Job drawing, mm, ordinate dimensions from the low corner. One solid piece. A direction names the side the tool comes from. Coordinates: 2 decimals unless noted, no trailing zeros. Order: outer loops, then holes, each group sorted by start corner. A loop starts at its lowest first (then second) coordinate and runs counter-clockwise, first axis right, second up. Notation, with made-up numbers: (56.25, 6.5) - (109.25, 6.5) arc R20 cw to (109.25, 25.5) - close; hole circle Ø6 at (-1.75, 29). An arc over 180 degrees is marked (long way). Return JSON: item names as keys, results as strings.
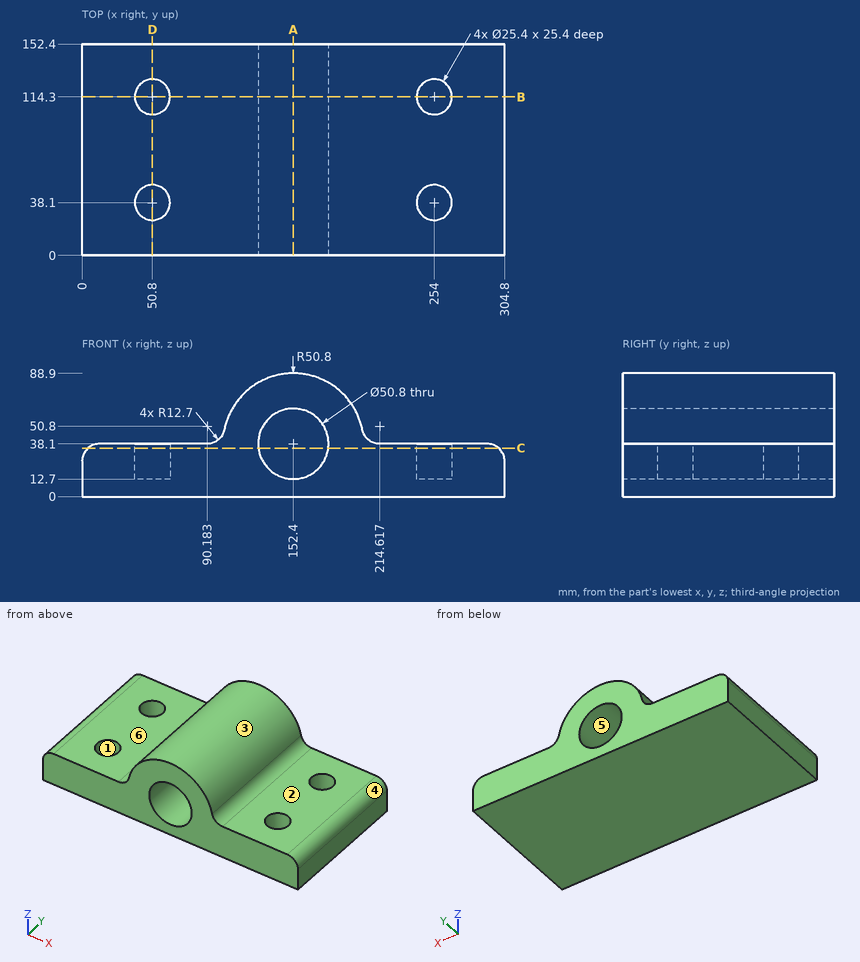
1. Drop flat-ended pins along their axis: pin 1 (12 mm diameter, centred on y = 49.5, z = 66.5, fed in from -X); pin 2 (12.5 mm diameter, centred on x = 252.5, y = 38, fed in from +Z); pin 3 (6 mm diameter, centred on y = 128, z = 58.5, fed in from -X). Give the stop position or say it passes through.
Check values:
{"pin 1": "x = 106.81", "pin 2": "z = 12.7", "pin 3": "x = 104.67"}
2. Probe L1, parallel to Y at x = 50, z = 25; L2, parallel to X at y = 104.5, z = 36 (1 decimal); L3, parallel to Z at x = 82.5, y = 60. List the from-to ranges inside material, lowest first.
Check values:
{"L1": "0 to 25.43, 50.77 to 101.63, 126.97 to 152.4", "L2": "5.7 to 42.7, 58.9 to 127.1, 177.7 to 245.9, 262.1 to 299.1", "L3": "0 to 38.1"}
3. Mould opens along X. For the marked faces 4, 5 and 6 say: pulls with the +X half, pulls with the -X half, needs draft (parallel to the pull), parting line crosses it, or undercut.
Check values:
{"face 4": "pulls with the +X half", "face 5": "undercut", "face 6": "needs draft"}
4. Cut at D-D on x = 50.8. Give the cut face in (y, z).
Check values:
{"outline": "(0, 0) - (152.4, 0) - (152.4, 38.1) - (127, 38.1) - (127, 12.7) - (101.6, 12.7) - (101.6, 38.1) - (50.8, 38.1) - (50.8, 12.7) - (25.4, 12.7) - (25.4, 38.1) - (0, 38.1) - close"}
5. Cut at A-A on x = 152.4. Give the cut face in (y, z), plus the area to 3 significant figures.
Check values:
{"outline": "(0, 0) - (152.4, 0) - (152.4, 12.7) - (0, 12.7) - close; (0, 63.5) - (152.4, 63.5) - (152.4, 88.9) - (0, 88.9) - close", "area": "5,810 mm²"}
6. Cut at B-B on y = 114.3. Give the cut face in (x, z), plus the area to 3 significant figures.
Check values:
{"outline": "(0, 0) - (304.8, 0) - (304.8, 25.4) arc R12.7 ccw to (292.1, 38.1) - (266.7, 38.1) - (266.7, 12.7) - (241.3, 12.7) - (241.3, 38.1) - (214.62, 38.1) arc R12.7 cw to (202.17, 48.26) arc R50.8 ccw to (102.63, 48.26) arc R12.7 cw to (90.18, 38.1) - (63.5, 38.1) - (63.5, 12.7) - (38.1, 12.7) - (38.1, 38.1) - (12.7, 38.1) arc R12.7 ccw to (0, 25.4) - close; hole circle Ø50.8 at (152.4, 38.1)", "area": "12,300 mm²"}
7. Cut at C-C on z = 35. Give the cut face in (x, y), plus the area to 3 significant figures.
Check values:
{"outline": "(4.39, 0) - (127.19, 0) - (127.19, 152.4) - (4.39, 152.4) - close; (177.61, 0) - (300.41, 0) - (300.41, 152.4) - (177.61, 152.4) - close; hole circle Ø25.4 at (50.8, 38.1); hole circle Ø25.4 at (50.8, 114.3); hole circle Ø25.4 at (254, 38.1); hole circle Ø25.4 at (254, 114.3)", "area": "35,400 mm²"}
8. Tool access for the marked faces 1, 2 and 3: list every direction of +Z, -Z, +X, -X, +Y, -Y with a clear straight run to the whole face (end or side of a thin tool).
Check values:
{"face 1": "+Z", "face 2": "+Z, +X, +Y, -Y", "face 3": "+Z, +Y, -Y"}
